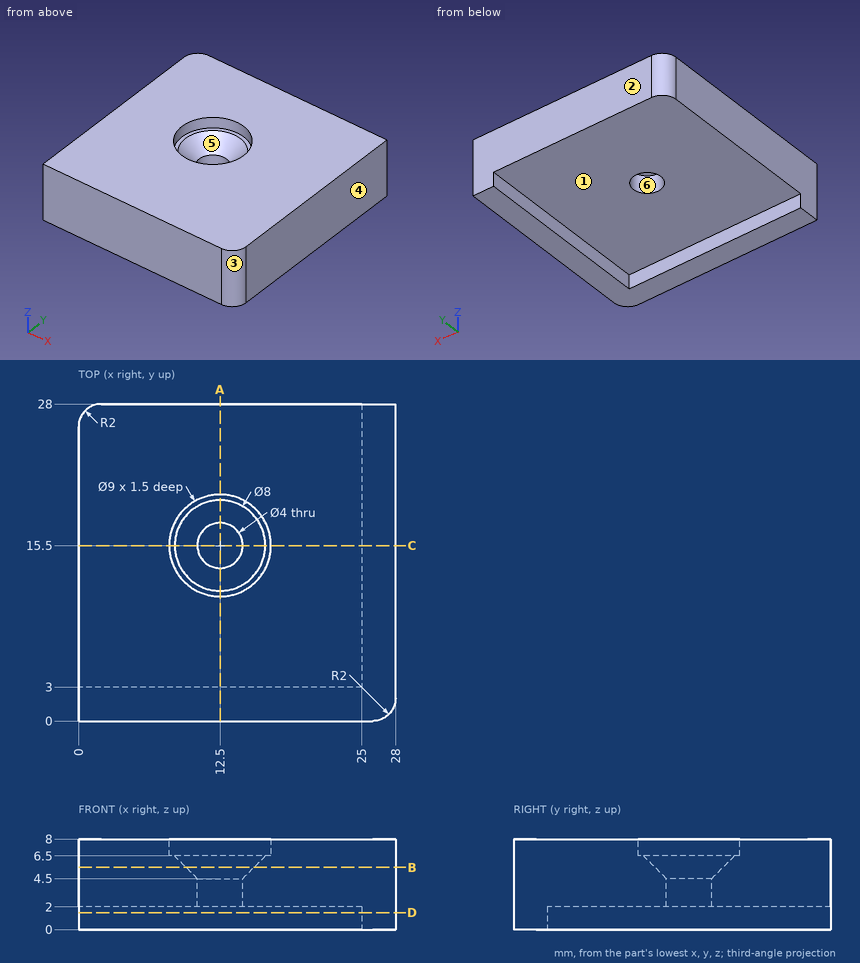
The drawing under review shows one solid part. Ordinate dimensions are in mm from its lowest x, y, z. A direction names the side the tool comes from. Coordinates: 2 decimals unless noted, no trailing zeros. Order: outer loops, then holes, each group sorted by start corner. A loop starts at its lowest first (then second) coordinate and runs counter-clockwise, first axis right, second up. Notation, with made-up numbers: M 38.25,14.25 L 66.25,14.25 A24 cw 66.25,49.25 Z; hole C 89,65 d4. An arc over 180 degrees is marked long. Use a Markdown table: item, result.
(1) Add section D-D (z = 1.5). Give the boundary of the cut face in (x, y), then the cut area to 3 significant figures.
Worked answers:
| item | result |
|---|---|
| outline | M 0,0 L 26,0 A2 ccw 28,2 L 28,28 L 25,28 L 25,3 L 0,3 Z |
| area | 158 mm2 |
(2) Wall thickness on probe 1 along X at (y, z) = (15.5, 3.25); probe 2 along Y at (x, z) = (12.5, 7.75); probe 3 along Z at (x, y) = (17.25, 13): over which ranges is each line inside the solid? List them lowest first.
Worked answers:
| item | result |
|---|---|
| probe 1 | x = 0 to 10.5, 14.5 to 28 |
| probe 2 | y = 0 to 11, 20 to 28 |
| probe 3 | z = 2 to 8 |
(3) For P1, Ø10.5, axis at x = 12.5, y = 15.5, coming from the -Z side; P2, Ø5, axis at x = 12.5, y = 15.5, coming from the +Z side, all flat-tipped, find the tip position at first contact; note any pin that passes through.
Worked answers:
| item | result |
|---|---|
| P1 | stops at z = 2 |
| P2 | stops at z = 5 |
(4) Add section B-B (z = 5.5). Give the boundary of the cut face in (x, y), then the cut area to 3 significant figures.
Worked answers:
| item | result |
|---|---|
| outline | M 0,0 L 26,0 A2 ccw 28,2 L 28,28 L 2,28 A2 ccw 0,26 Z; hole C 12.5,15.5 d6 |
| area | 754 mm2 |
(5) Add section C-C (y = 15.5). Give the boundary of the cut face in (x, z).
Worked answers:
| item | result |
|---|---|
| outline | M 0,2 L 10.5,2 L 10.5,4.5 L 8.5,6.5 L 8,6.5 L 8,8 L 0,8 Z; M 14.5,2 L 25,2 L 25,0 L 28,0 L 28,8 L 17,8 L 17,6.5 L 16.5,6.5 L 14.5,4.5 Z |
(6) For the marked faces 1 and 2, list the 3-axis set-ups (+Z, -Z, +X, -X, +Y, -Y) from which the entire face can be reached by the end or side of a thin tool; tool diameter is ignored.
Worked answers:
| item | result |
|---|---|
| face 1 | -Z, -X, +Y |
| face 2 | +Z, -Z, +X, -X, +Y |
(7) Draft analysis for pull direction Y (two halves, no side actions). For the marked faces 3, 4, 5 and 6, state which applies: released by +Y, released by -Y, zero draft, split by the parting line, or undercut.
Worked answers:
| item | result |
|---|---|
| face 3 | released by -Y |
| face 4 | zero draft |
| face 5 | undercut |
| face 6 | undercut |
(8) Add section A-A (x = 12.5). Give the boundary of the cut face in (y, z), then the cut area to 4 significant figures.
Worked answers:
| item | result |
|---|---|
| outline | M 0,0 L 3,0 L 3,2 L 13.5,2 L 13.5,4.5 L 11.5,6.5 L 11,6.5 L 11,8 L 0,8 Z; M 17.5,2 L 28,2 L 28,8 L 20,8 L 20,6.5 L 19.5,6.5 L 17.5,4.5 Z |
| area | 138.5 mm2 |
